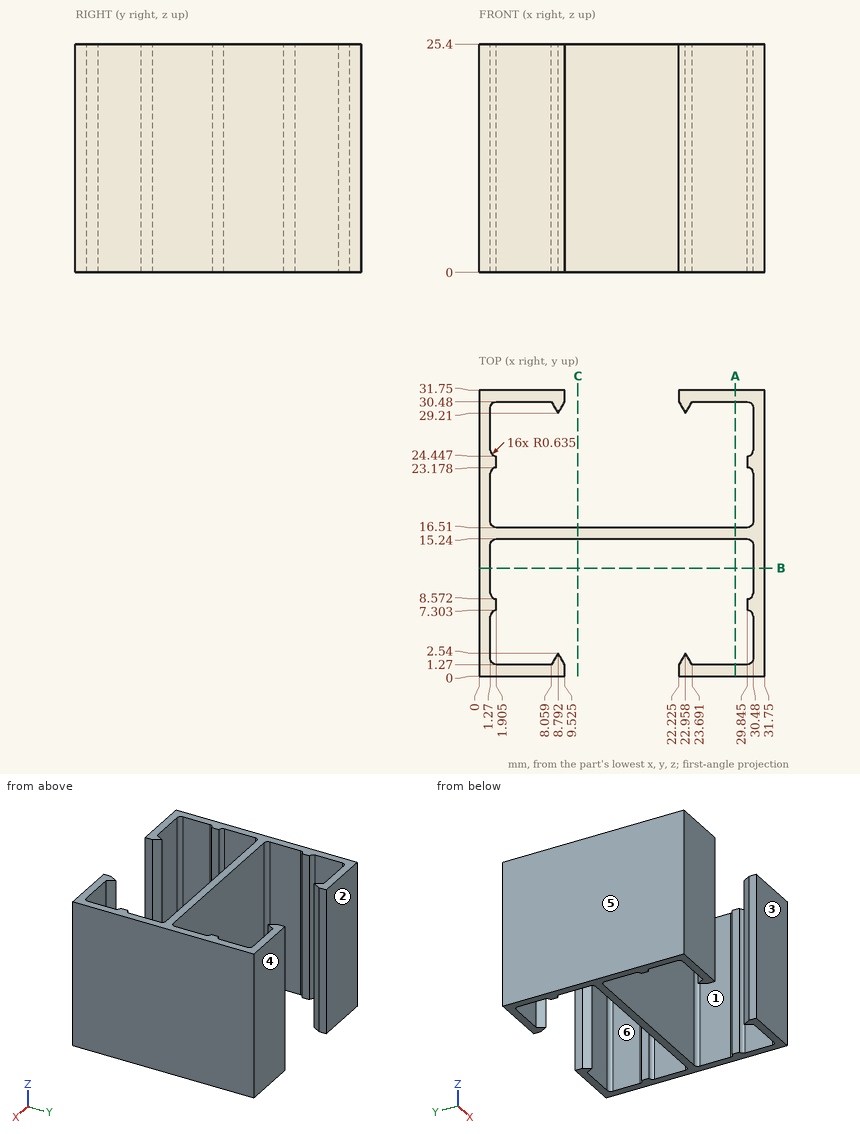
Verification items for this drawing (mm, ordinates from the low corner). A direction names the side the tool comes from. Coordinates: 2 decimals unless noted, no trailing zeros. Loops run counter-clockwise (first coordinate to the right, second up) from the corner with the lowest first, then second, coordinate; pieces in that order, holes last. Notation, with made-up numbers: (77, -5) - (89, -5) arc R22 cw to (89, 34) - close; hole circle Ø7 at (21.5, -18.5). An arc over 180 degrees is marked (long way). Use one line per item in the form item = value. Start each with the question number.
Item 1: Mould release check, pull along Y, two halves, no side actions. Record for the marked faces 3, 4, 5 and 6: +Y half, -Y half, draft (parallel to the pull), parting line (faces both ways), or undercut.
Item 2: Section check C-C, the plane x = 11. Enter the section's corners in (y, z).
Item 3: Gauge pin test, flat ends, axial feed: pin 1 (6 mm diameter, centred on y = 11.5, z = 16.5, fed in from -X); pin 2 (2 mm diameter, centred on x = 11, z = 9, fed in from -Y). Record the tip position at first contact, or that the pin passes through.
Item 4: Thickness scan on probe 1 along Y at (x, z) = (5, 17); probe 2 along X at (y, z) = (26.5, 18.5); probe 3 along Y at (x, z) = (22, 16). Record the ranges inside material, lowest first.
Item 5: Section check A-A, the plane x = 28.5. Enter the section's corners in (y, z).
Item 6: Tool access check on the marked faces 1 and 2. Record the directions out of +Z, -Z, +X, -X, +Y, -Y that give a thin tool (end or side, any length) a straight path to the whole face; none if there is none.
Item 7: Section check B-B, the plane y = 12. Enter the section's corners in (x, z).
Computed:
q1.face_3 = -Y half
q1.face_4 = +Y half
q1.face_5 = draft
q1.face_6 = undercut
q2.outline = (15.24, 0) - (16.51, 0) - (16.51, 25.4) - (15.24, 25.4) - close
q3.pin_1 = 0
q3.pin_2 = 15.24
q4.probe_1 = 0 to 1.27, 15.24 to 16.51, 30.48 to 31.75
q4.probe_2 = 0 to 1.27, 30.48 to 31.75
q4.probe_3 = 15.24 to 16.51
q5.outline = (0, 0) - (1.27, 0) - (1.27, 25.4) - (0, 25.4) - close; (15.24, 0) - (16.51, 0) - (16.51, 25.4) - (15.24, 25.4) - close; (30.48, 0) - (31.75, 0) - (31.75, 25.4) - (30.48, 25.4) - close
q6.face_1 = +Z, -Z
q6.face_2 = +Z, -Z, +X, -X, +Y
q7.outline = (0, 0) - (1.27, 0) - (1.27, 25.4) - (0, 25.4) - close; (30.48, 0) - (31.75, 0) - (31.75, 25.4) - (30.48, 25.4) - close
